from build123d import *

# Parameters (mm, degrees)
F1_DEPTH  = 14
F2_R      = 2
F0_W      = 70
F0_H      = 80
F3_DEPTH  = 13.9
F4_W      = 7.4
F4_H      = 4
F4_H_2    = 81
F5_DEPTH  = 4
F6_R      = 1
F7_W      = 3
F7_H      = 10
F8_DEPTH  = 3
F9_DEPTH  = 2.25
F11_DEPTH = 3
F10_R     = 1.75
F12_DEPTH = 2.5


with BuildPart() as f1:
    # F0 (on Front) → F1 (new body)
    with BuildSketch(Plane.XZ):
        Polygon((0, 100), (0, 0), (85, 0), (85, 10), (15, 10), (15, 90), (85, 90), (85, 100), align=None)
    extrude(amount=F1_DEPTH)

    # F2
    f2_edges = [f1.edges().sort_by_distance(p)[0] for p in [
        (42.5, -14, 100),
        (42.5, 0, 100),
        (42.5, -14, 0),
        (42.5, 0, 0),
    ]]
    fillet(f2_edges, radius=F2_R)

    # F0 (on Front) → F3 (join)
    with BuildSketch(Plane.XZ):
        with Locations((50, 50)):
            Rectangle(F0_W, F0_H)
    extrude(amount=F3_DEPTH)

    # F4 (on face) → F5 (cut)
    with BuildSketch(Plane(origin=(0, 0, 0), x_dir=(0, -1, 0), z_dir=(-1, 0, 0))):
        with BuildLine():
            Line((12, 100), (10.7, 100))
            Line((10.7, 100), (10.7, 96))
            Line((10.7, 96), (14, 96))
            Line((14, 96), (14, 98))
            ThreePointArc((14, 98), (13.4142135624, 99.4142135624), (12, 100))
        make_face()
        with Locations((7, 98)):
            Rectangle(F4_W, F4_H)
        with BuildLine():
            Line((3.3, 96), (3.3, 100))
            Line((3.3, 100), (2, 100))
            ThreePointArc((2, 100), (0.5857864376, 99.4142135624), (0, 98))
            Line((0, 98), (0, 96))
            Line((0, 96), (3.3, 96))
        make_face()
        with Locations((7, 55.5)):
            Rectangle(F4_W, F4_H_2)
    extrude(amount=-F5_DEPTH, mode=Mode.SUBTRACT)

    # F6
    f6_edges = [f1.edges().sort_by_distance(p)[0] for p in [
        (4, -1.65, 96),
        (4, -12.35, 96),
    ]]
    fillet(f6_edges, radius=F6_R)

    # F7 (on face) → F8 (cut)
    with BuildSketch(Plane.XZ):
        with BuildLine():
            Line((82, 10.8), (82, 10))
            Line((82, 10), (85, 10))
            Line((85, 10), (85, 12))
            Line((85, 12), (83.2, 12))
            ThreePointArc((83.2, 12), (82.3514718626, 11.6485281374), (82, 10.8))
        make_face()
        with Locations((83.5, 5)):
            Rectangle(F7_W, F7_H)
    extrude(amount=F8_DEPTH, mode=Mode.SUBTRACT)

    # F7 (on face) → F9 (cut)
    with BuildSketch(Plane.XZ):
        with BuildLine():
            Line((35.7679491924, 10), (78.2320508076, 10))
            ThreePointArc((78.2320508076, 10), (78.245506934, 10.1246782406), (78.25, 10.25))
            ThreePointArc((78.25, 10.25), (77.7374368671, 11.4874368671), (76.5, 12))
            Line((76.5, 12), (37.5, 12))
            ThreePointArc((37.5, 12), (36.2625631329, 11.4874368671), (35.75, 10.25))
            ThreePointArc((35.75, 10.25), (35.754493066, 10.1246782406), (35.7679491924, 10))
        make_face()
        with BuildLine():
            ThreePointArc((76.5, 8.5), (77.6456439237, 8.9271243445), (78.2320508076, 10))
            Line((78.2320508076, 10), (35.7679491924, 10))
            ThreePointArc((35.7679491924, 10), (36.3543560763, 8.9271243445), (37.5, 8.5))
            Line((37.5, 8.5), (76.5, 8.5))
        make_face()
    extrude(amount=F9_DEPTH, mode=Mode.SUBTRACT)

    # F10 (on face) → F11 (cut)
    with BuildSketch(Plane(origin=(0, 0, 0), x_dir=(1, 0, 0), z_dir=(0, 0, -1))):
        with BuildLine():
            Line((83.25, 6), (85, 6))
            Line((85, 6), (85, 8.5))
            Line((85, 8.5), (83.25, 8.5))
            ThreePointArc((83.25, 8.5), (82.3661165235, 8.1338834765), (82, 7.25))
            ThreePointArc((82, 7.25), (82.3661165235, 6.3661165235), (83.25, 6))
        make_face()
    extrude(amount=-F11_DEPTH, mode=Mode.SUBTRACT)

    # F10 (on face) → F12 (cut)
    with BuildSketch(Plane(origin=(0, 0, 0), x_dir=(1, 0, 0), z_dir=(0, 0, -1))):
        with Locations((66.9, 7.25)):
            Circle(F10_R)
    extrude(amount=-F12_DEPTH, mode=Mode.SUBTRACT)

    # F13: F1 across face


with BuildPart() as f1_1:
    add(f1.part)
    add(f1.part.mirror(Plane(origin=(85, -7.100228209, 51.4155420461), x_dir=(0, 1, 0), z_dir=(1, 0, 0))))


solid = f1_1.part
Geometry: final body of the model. Coordinates: model frame, mm. A direction names the side the tool comes from. Coordinates: 2 decimals unless noted, no trailing zeros. Loops run counter-clockwise (first coordinate to the right, second up) from the corner with the lowest first, then second, coordinate; pieces in that order, holes last. Notation, with made-up numbers: (82, 75.25) - (141, 75.25) arc R14 ccw to (141, 90.25) - close; hole circle Ø8 at (40.25, 18.25). An arc over 180 degrees is marked (long way). Put each result on its own line as item: value. Start each with the question number.
Q1. Pull-direction query (X, two-part tool) for faces 6 (the flat face through (170, -2, 49)), 7 (the cylindrical face through (65.15, -7.33, 1.23)), 8 (the flat face through (85, -8.5, 1)); classes: released by +X, released by -X, zero draft, split by the parting line, or undercut.
Q2. Cut plane B-B, the plane x = 66.9. Return loops of the section in (y, z).
Q3. Cut plane A-A, the plane z = 70.5. Return loops of the section in (x, y), and give its area (3 significant figures).
Q4. Set-up query: faces 1 (the flat face through (166, -7, 58)), 2 (the flat face through (113, -2.25, 10)), 3 (the flat face through (169, -2, 96)), 4 (the flat face through (85, -3, 6)), 5 (the flat face through (1, -2, 96)). Return all of +Z, -Z, +X, -X, +Y, -Y with unobstructed straight access to the full face (end or side cutting, diameter ignored); none if empty.
Q5. Pin query (flat end, axial travel): pin 1 Ø2 at (y, z) = (-4.5, 79.5) entering from +X; pin 2 Ø1.5 at (x, z) = (84, 1) entering from +Y; pin 3 Ø1.1 at (x, y) = (57, -1) entering from -Z. Return the tip coordinate at first contact, or that it passes through.
Q6. Line query: line 1 (X direction, y = -7.25, z = 1.35); line 2 (Z direction, x = 125, y = -1.75); line 3 (X direction, y = -4.25, z = 49.5). Output: solid intervals per line, ascending.
Filled sheet:
1. face 6: released by +X
1. face 7: undercut
1. face 8: undercut
2. outline: (-14, 2) arc R2 ccw to (-12, 0) - (-9, 0) - (-9, 2.5) - (-5.5, 2.5) - (-5.5, 0) - (-2, 0) arc R2 ccw to (0, 2) - (0, 8.5) - (-2.25, 8.5) - (-2.25, 12) - (0, 12) - (0, 98) arc R2 ccw to (-2, 100) - (-12, 100) arc R2 ccw to (-14, 98) - (-14, 90) - (-13.9, 90) - (-13.9, 10) - (-14, 10) - close
3. outline: (0, -14) - (15, -14) - (15, -13.9) - (155, -13.9) - (155, -14) - (170, -14) - (170, -10.7) - (166, -10.7) - (166, -3.3) - (170, -3.3) - (170, 0) - (0, 0) - (0, -3.3) - (4, -3.3) - (4, -10.7) - (0, -10.7) - close
3. area: 2,310 mm²
4. face 1: +Z, +X
4. face 2: +Y
4. face 3: +Z, +X, +Y, -Y
4. face 4: -Z, +Y
4. face 5: +Z, -X, +Y, -Y
5. pin 1: x = 166
5. pin 2: y = -3
5. pin 3: z = 0.05
6. line 1: 0 to 65.15, 68.65 to 82, 88 to 101.35, 104.85 to 170
6. line 2: 0.02 to 8.5, 12 to 99.98
6. line 3: 4 to 166
